The listing builds one solid part. Answer for the finished solid, in the listing's coordinates (mm). A direction names the side the tool comes from. Round coordinates to 2 decimals unless told otherwise and drop trailing zeros. Loops run counter-clockwise (first coordinate to the right, second up) from the corner with the lowest first, then second, coordinate; pieces in that order, holes last. Notation, with made-up numbers: M 15,-14 L 39,-14 A24 ccw 39,6 Z; hole C -29,-36.5 d5. An arc over 180 degrees is marked long. Put each result on its own line as item: value. Start each with the question number.
(1) Section B-B, the plane x = 0 is taken. Determine the outline of the cut face in (y, z) (3 decimals), then the cut area to 3 significant figures.
(2) Determine the mould class of faces 6 (the face through (20.064, 3.219, -47.663)), 7 (the face through (23, -21.59, -29)), 8 (the face through (0.954, 5.009, -55.646)) for opening direction X: released by +X, released by -X, zero draft, split by the parting line, or undercut.
(3) Which of the six approach directions +Z, -Z, +X, -X, +Y, -Y give full straight-line access (tool end or side, diameter ignored) to faces 1 (the face through (25.4, -12, -30)), 2 (the face through (23, -12, -16.637)), 3 (the face through (38.28, 3.13, -55.57)), 4 (the face through (34, 2.54, -30)), 5 (the face through (-11.976, 5.151, -49.151))?
(4) Flat-ended cylindrical pins translate along their axes: P1, Ø4, axis at x = 18.415, z = -0.762, coming from the -Y side; P2, Ø10, axis at y = -6, z = -4, coming from the -X side; P3, Ø16.5, axis at x = 38.5, z = -28.5, coming from the +Y side; P4, Ø3, axis at x = 30.5, y = 4, coming from the +Z side. Find the tip coordinate at first contact, or state that the pin passes through.
(5) Section C-C, the plane z = 0 is taken. Determine the outline of the cut face in (x, y) (3 decimals).
(6) Section D-D, the plane y = 1.5 is taken. Determine the outline of the cut face in (x, z) (3 decimals).
(7) Straight lines are drawn through the part: line 1 (X direction, y = -13.5, z = -42); line 2 (Z direction, x = 25, y = 3); line 3 (Y direction, x = 22.5, z = -14). For each, find the intervals that lie inside material, in ascending order.
(8) Section A-A, the plane x = 13.5 is taken. Determine the outline of the cut face in (y, z).
```python
from build123d import *

# Parameters (mm, degrees)
SKETCH1_W                = 38.1
SKETCH1_H                = 69.85
SKETCH1_R                = 3.175
SKETCH1_W_2              = 25.4
SKETCH1_H_2              = 35.56
BOSS_EXTRUDE1_DEPTH      = 6.35
SKETCH2_W                = 27.432
SKETCH2_H                = 25.4
CUT_EXTRUDE1_DEPTH       = 3.81
SKETCH3_W                = 33.528
SKETCH3_H                = 38.1
CUT_EXTRUDE2_DEPTH       = 83.161835082
SKETCH9_W                = 4.572
SKETCH9_H                = 25.4
BOSS_EXTRUDE5_DEPTH      = 21.59
BOSS_EXTRUDE6_DEPTH      = 3.81
BOSS_EXTRUDE6_DEPTH_BACK = 0.000254
SKETCH10_W               = 38.1
SKETCH10_H               = 15.875
SKETCH10_R               = 3.175
CUT_EXTRUDE4_DEPTH       = 88.853896578
CUT_EXTRUDE4_DEPTH_BACK  = 10.16
SKETCH11_R               = 1.651
FILLET4_R                = 2.54
CHAMFER3_SIZE            = 1.905


with BuildPart() as part:
    # Sketch1 → Boss-Extrude1 (new body)
    # profile 1 of 4: a face of its own
    with BuildSketch(Plane(origin=(0, 0, 0), x_dir=(1, 0, 0), z_dir=(0, 1, 0))):
        with Locations((6.35, 29.337)):
            Rectangle(SKETCH1_W, SKETCH1_H)
        with Locations(Location((0, 58.674, 0), (0, 0, 270))):
            Circle(SKETCH1_R, mode=Mode.SUBTRACT)
        with Locations(Location((0, 0, 0), (0, 0, 270))):
            Circle(SKETCH1_R, mode=Mode.SUBTRACT)
    # profile 2 of 4: a face of its own
    with BuildSketch(Plane(origin=(0, 0, 0), x_dir=(1, 0, 0), z_dir=(0, 1, 0))):
        Polygon((25.4, 47.117), (50.8, 47.117), (25.4, 64.262), align=None)
    # profile 3 of 4: a face of its own
    with BuildSketch(Plane(origin=(0, 0, 0), x_dir=(1, 0, 0), z_dir=(0, 1, 0))):
        with Locations((38.1, 29.337)):
            Rectangle(SKETCH1_W_2, SKETCH1_H_2)
    # profile 4 of 4: a face of its own
    with BuildSketch(Plane(origin=(0, 0, 0), x_dir=(1, 0, 0), z_dir=(0, 1, 0))):
        Polygon((25.4, -5.588), (50.8, 11.557), (25.4, 11.557), align=None)
    extrude(amount=BOSS_EXTRUDE1_DEPTH)

    # Sketch2 → Cut-Extrude1 (cut)
    with BuildSketch(Plane(origin=(0, 6.35, 0), x_dir=(1, 0, 0), z_dir=(0, 1, 0))):
        with Locations((34.544, 29.337)):
            Rectangle(SKETCH2_W, SKETCH2_H)
    extrude(amount=-CUT_EXTRUDE1_DEPTH, mode=Mode.SUBTRACT)

    # Sketch3 → Cut-Extrude2 (cut, through all)
    with BuildSketch(Plane(origin=(0, 6.35, 0), x_dir=(1, 0, 0), z_dir=(0, 1, 0))):
        with Locations((4.064, 29.337)):
            Rectangle(SKETCH3_W, SKETCH3_H)
    extrude(amount=-CUT_EXTRUDE2_DEPTH, mode=Mode.SUBTRACT)

    # Sketch9 → Boss-Extrude5 (add)
    with BuildSketch(Plane.XZ):
        with Locations((23.114, -29.337)):
            Rectangle(SKETCH9_W, SKETCH9_H)
    extrude(amount=BOSS_EXTRUDE5_DEPTH)

    # Sketch10 → Boss-Extrude6 (add, two sides: drawn at the far end of the back side and taken through both)
    # profile 1 of 2: a face of its own
    with BuildSketch(Plane(origin=(0, 6.35, 0), x_dir=(1, 0, 0), z_dir=(0, 1, 0)).offset(-BOSS_EXTRUDE6_DEPTH_BACK)):
        with Locations((6.35, 56.3245)):
            Rectangle(SKETCH10_W, SKETCH10_H)
        with Locations(Location((0, 58.674, 0), (0, 0, 270))):
            Circle(SKETCH10_R, mode=Mode.SUBTRACT)
    # profile 2 of 2: a face of its own
    with BuildSketch(Plane(origin=(0, 6.35, 0), x_dir=(1, 0, 0), z_dir=(0, 1, 0)).offset(-BOSS_EXTRUDE6_DEPTH_BACK)):
        with Locations((6.35, 2.3495)):
            Rectangle(SKETCH10_W, SKETCH10_H)
        with Locations(Location((0, 0, 0), (0, 0, 270))):
            Circle(SKETCH10_R, mode=Mode.SUBTRACT)
    extrude(amount=BOSS_EXTRUDE6_DEPTH + BOSS_EXTRUDE6_DEPTH_BACK)

    # Sketch11 → Cut-Extrude4 (cut, two sides: drawn at the far end of the back side and taken through both)
    with BuildSketch(Plane(origin=(0, 10.16, 0), x_dir=(1, 0, 0), z_dir=(0, 1, 0)).offset(-CUT_EXTRUDE4_DEPTH_BACK)):
        with Locations(Location((18.415, 57.912, 0), (0, 0, 90))):
            Circle(SKETCH11_R)
        with Locations(Location((18.415, 0.762, 0), (0, 0, 90))):
            Circle(SKETCH11_R)
    extrude(amount=CUT_EXTRUDE4_DEPTH + CUT_EXTRUDE4_DEPTH_BACK, mode=Mode.SUBTRACT)

    # Fillet4
    fillet4_edges = [part.edges().sort_by_distance(p)[0] for p in [
        (-12.7, 5.08, 5.588),
        (-12.7, 5.08, -64.262),
        (20.828, 3.175, -48.387),
        (-12.7, 5.08, -10.287),
        (-12.7, 5.08, -48.387),
        (20.828, 3.175, -10.287),
    ]]
    fillet(fillet4_edges, radius=FILLET4_R)

    # Chamfer3
    chamfer3_edges = [part.edges().sort_by_distance(p)[0] for p in [
        (23.114, 0, -42.037),
        (25.4, 0, -29.337),
        (23.114, 0, -16.637),
    ]]
    chamfer(chamfer3_edges, length=CHAMFER3_SIZE)


solid = part.part
```
Recorded:
1. outline: M 0,-64.262 L 10.16,-64.262 L 10.16,-61.849 L 0,-61.849 Z; M 0,-55.499 L 10.16,-55.499 L 10.16,-48.387 L 0,-48.387 Z; M 0,-10.287 L 10.16,-10.287 L 10.16,-3.175 L 0,-3.175 Z; M 0,3.175 L 10.16,3.175 L 10.16,5.588 L 0,5.588 Z
1. area: 194 mm²
2. face 6: released by -X
2. face 7: zero draft
2. face 8: undercut
3. face 1: +Z, -Z, +X, -Y
3. face 2: +Z, +X, -X, -Y
3. face 3: -Z, +X, +Y, -Y
3. face 4: -X, +Y
3. face 5: -X, +Y, -Y
4. P1: stops at y = 0
4. P2: passes through
4. P3: stops at y = 2.54
4. P4: stops at z = 3.16
5. outline: M -12.7,0 L -3.175,0 L -3.175,10.16 L -12.7,10.16 Z; M 3.175,0 L 16.95,0 L 16.95,10.16 L 3.175,10.16 Z; M 19.88,0 L 33.679,0 L 33.679,6.35 L 25.4,6.35 L 25.4,10.16 L 19.88,10.16 Z
6. outline: M -12.7,-61.722 A2.54 ccw -10.16,-64.262 L 25.4,-64.262 L 50.8,-47.117 L 50.8,-11.557 L 25.4,5.588 L -10.16,5.588 A2.54 ccw -12.7,3.048 L -12.7,-7.747 A2.54 ccw -10.16,-10.287 L 18.288,-10.287 A2.54 cw 20.828,-12.827 L 20.828,-45.847 A2.54 cw 18.288,-48.387 L -10.16,-48.387 A2.54 ccw -12.7,-50.927 Z; hole C 0,-58.674 d6.35; hole C 0,0 d6.35; hole C 18.415,-57.912 d3.302; hole C 18.415,-0.762 d3.302
7. line 1: x = 20.83 to 25.4
7. line 2: z = -64.26 to -42.04, -16.64 to 5.59
7. line 3: y = 0 to 6.35
8. outline: M 0,-64.26 L 10.16,-64.26 L 10.16,-48.39 L 0,-48.39 Z; M 0,-10.29 L 10.16,-10.29 L 10.16,5.59 L 0,5.59 Z
